Could you check a few things on this model? Use its own coordinates, in mm. A direction names the side the tool comes from. Round coordinates to 2 decimals unless told otherwise and drop trailing zeros. Loops run counter-clockwise (first coordinate to the right, second up) from the corner with the lowest first, then second, coordinate; pieces in that order, holes last. Notation, with made-up numbers: M -22,88 L 37,88 A13 ccw 37,106 Z; hole C -2.75,41.5 d6. An arc over 180 degrees is marked long. Answer in a Markdown table with one row per item.
```python
from build123d import *

# Parameters (mm, degrees)
SKETCH1_W           = 76.2
SKETCH1_H           = 25.4
BOSS_EXTRUDE1_DEPTH = 3.175


with BuildPart() as part:
    # Sketch1 → Boss-Extrude1 (new body)
    with BuildSketch(Plane(origin=(0, 0, 0), x_dir=(1, 0, 0), z_dir=(0, 1, 0))):
        Rectangle(SKETCH1_W, SKETCH1_H)
        with BuildLine():
            Line((-23.3553, 5.2197), (-14.7447, 5.2197))
            ThreePointArc((-14.7447, 5.2197), (-9.525, 0), (-14.7447, -5.2197))
            Line((-14.7447, -5.2197), (-23.3553, -5.2197))
            ThreePointArc((-23.3553, -5.2197), (-28.575, 0), (-23.3553, 5.2197))
        make_face(mode=Mode.SUBTRACT)
        with BuildLine():
            Line((23.3553, 5.2197), (14.7447, 5.2197))
            ThreePointArc((14.7447, 5.2197), (9.525, 0), (14.7447, -5.2197))
            Line((14.7447, -5.2197), (23.3553, -5.2197))
            ThreePointArc((23.3553, -5.2197), (28.575, 0), (23.3553, 5.2197))
        make_face(mode=Mode.SUBTRACT)
    extrude(amount=BOSS_EXTRUDE1_DEPTH)


solid = part.part
```
1) I want a section at A-A, the plane z = 0. Please give me the cut outline in (x, y) (3 decimals), plus the area to 3 significant figures.
Computed:
| item | result |
|---|---|
| outline | M -38.1,0 L -28.575,0 L -28.575,3.175 L -38.1,3.175 Z; M -9.525,0 L 9.525,0 L 9.525,3.175 L -9.525,3.175 Z; M 28.575,0 L 38.1,0 L 38.1,3.175 L 28.575,3.175 Z |
| area | 121 mm² |
2) I need wall thicknesses on line 1 (X direction, y = 2.4, z = 2); line 2 (Z direction, x = 21, y = 1.9); line 3 (X direction, y = 2.8, z = -4.5). Which ranges of each line are inside material? Lowest first, please.
Computed:
| item | result |
|---|---|
| line 1 | x = -38.1 to -28.18, -9.92 to 9.92, 28.18 to 38.1 |
| line 2 | z = -12.7 to -5.22, 5.22 to 12.7 |
| line 3 | x = -38.1 to -26, -12.1 to 12.1, 26 to 38.1 |
3) If we mould it in two halves opening along Z, with no side actions, what happens to faces 1 (the face through (-28.574, 1.565, 0.115)), 2 (the face through (38.1, 2, 0)), 3 (the face through (-1, 2, -12.7))? For each: released by +Z, released by -Z, zero draft, split by the parting line, or undercut.
Computed:
| item | result |
|---|---|
| face 1 | undercut |
| face 2 | zero draft |
| face 3 | released by -Z |
4) I want a section at D-D, the plane z = -4.5. Please give me the cut outline in (x, y) (3 decimals), plus the area to 3 significant figures.
Computed:
| item | result |
|---|---|
| outline | M -38.1,0 L -26,0 L -26,3.175 L -38.1,3.175 Z; M -12.1,0 L 12.1,0 L 12.1,3.175 L -12.1,3.175 Z; M 26,0 L 38.1,0 L 38.1,3.175 L 26,3.175 Z |
| area | 154 mm² |
5) I want a section at C-C, the plane x = 22. Please give me the cut outline in (y, z) (3 decimals).
Computed:
| item | result |
|---|---|
| outline | M 0,-12.7 L 3.175,-12.7 L 3.175,-5.22 L 0,-5.22 Z; M 0,5.22 L 3.175,5.22 L 3.175,12.7 L 0,12.7 Z |
6) I want a section at B-B, the plane y = 1.3. Please give me the cut outline in (x, z), plus the area to 3 significant figures.
Computed:
| item | result |
|---|---|
| outline | M -38.1,-12.7 L 38.1,-12.7 L 38.1,12.7 L -38.1,12.7 Z; hole M -23.36,-5.22 L -14.74,-5.22 A5.22 ccw -14.74,5.22 L -23.36,5.22 A5.22 ccw Z; hole M 14.74,-5.22 L 23.36,-5.22 A5.22 ccw 23.36,5.22 L 14.74,5.22 A5.22 ccw Z |
| area | 1,580 mm² |
7) Which directions (+Z, -Z, +X, -X, +Y, -Y) give clear straight access to the entire face, cutting with the end or side of a thin tool? Please do faces 4 (the face through (19, 2, -5.22)), 5 (the face through (-1, 0, 0)).
Computed:
| item | result |
|---|---|
| face 4 | +Y, -Y |
| face 5 | +Z, -Z, +X, -X, -Y |
